```python
from build123d import *

# Parameters (mm, degrees)
BOX002_W          = 10
BOX002_H          = 8
BOX002_DEPTH      = 5
CYLINDER003_R     = 2
CYLINDER003_DEPTH = 10
ARRAY003_X_COUNT  = 5
ARRAY003_X_PITCH  = 10
ARRAY003_Z_COUNT  = 2
ARRAY003_Z_PITCH  = 8
BOX001_W          = 57
BOX001_H          = 2
BOX001_DEPTH      = 22.3


with BuildPart() as cube:
    # Box002 → Box002 (new body)
    with BuildSketch(Plane(origin=(-15, -27, -2.5), x_dir=(1, 0, 0), z_dir=(0, 0, 1))):
        with Locations((5, 4)):
            Rectangle(BOX002_W, BOX002_H)
    extrude(amount=BOX002_DEPTH)


with BuildPart() as array003:
    # Cylinder003 → Cylinder003 (new body)
    with BuildSketch(Plane(origin=(-30, -16, 7), x_dir=(1, 0, 0), z_dir=(0, -1, 0))):
        Circle(CYLINDER003_R)
    extrude(amount=CYLINDER003_DEPTH)

    # Array003 X: Array003 ×5


with BuildPart() as array003_1:
    add(array003.part)
    with Locations(*[(i * ARRAY003_X_PITCH, 0, 0) for i in range(1, ARRAY003_X_COUNT)]):
        add(array003.part)

    # Array003 Z: Array003 ×2


with BuildPart() as array003_2:
    add(array003_1.part)
    with Locations(*[(0, 0, i * ARRAY003_Z_PITCH) for i in range(1, ARRAY003_Z_COUNT)]):
        add(array003_1.part)


with BuildPart() as cut006:
    # Box001 → Box001 (new body)
    with BuildSketch(Plane(origin=(-38.5, -22, 0), x_dir=(1, 0, 0), z_dir=(0, 0, 1))):
        with Locations((28.5, 1)):
            Rectangle(BOX001_W, BOX001_H)
    extrude(amount=BOX001_DEPTH)

    # Cut005: cut Array003
    add(array003_2.part, mode=Mode.SUBTRACT)

    # Cut006: cut Cube
    add(cube.part, mode=Mode.SUBTRACT)


solid = cut006.part
```
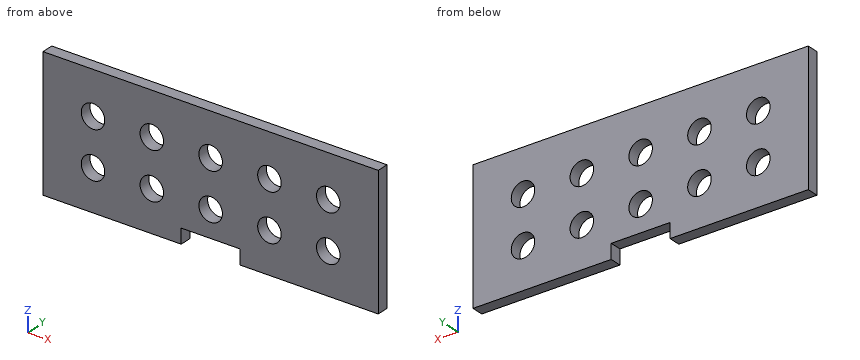
CAD build for the part. Positions are in the model's coordinates, mm. Round coordinates to 2 decimals unless told otherwise and drop trailing zeros. Write each loop counter-clockwise with the first axis right and the second up, starting at its lowest first coordinate (ties: lowest second). Pieces come first, ordered by that corner, then holes. Notation, with made-up numbers: (-23, 1.25) -> (-2, 1.25) arc R14 cw to (-2, 16.25) -> close; hole circle Ø6 at (84.5, 3). An arc over 180 degrees is marked (long way). Answer in a Markdown table with one row per item. Add a question column.
Item 1: Saw through at B-B, the plane y = -20.6. Count the separate pieces of the cut face and the enclosed holes in it, then the cut area to 3 significant figures.
Item 2: Saw through at A-A, the plane z = 15. Write the cut outline in (x, y), then the cut area to 3 significant figures.
Item 3: Saw through at D-D, the plane x = -0.5. Write the cut outline in (y, z).
Item 4: Drop a flat-ended pin along its axis: pin 1 Ø2 at (x, z) = (-20.5, 15) entering from +Y. Give the stop position or say it passes through.
Item 5: Drill centre lines: line 1 (X direction, y = -21.45, z = 15); line 2 (Z direction, x = -20, y = -21.5); line 3 (Z direction, x = -10, y = -20.7). Where is each one in solid material? Low to high. Write a range as from..to.
Item 6: Saw through at C-C, the plane x = -20. Write the cut outline in (y, z), then the cut area to 3 significant figures.
Findings below:
| question | item | result |
|---|---|---|
| 1 | separate pieces | 1 |
| 1 | enclosed holes | 10 |
| 1 | area | 1,120 mm^2 |
| 2 | outline | (-38.5, -22) -> (-32, -22) -> (-32, -20) -> (-38.5, -20) -> close; (-28, -22) -> (-22, -22) -> (-22, -20) -> (-28, -20) -> close; (-18, -22) -> (-12, -22) -> (-12, -20) -> (-18, -20) -> close; (-8, -22) -> (-2, -22) -> (-2, -20) -> (-8, -20) -> close; (2, -22) -> (8, -22) -> (8, -20) -> (2, -20) -> close; (12, -22) -> (18.5, -22) -> (18.5, -20) -> (12, -20) -> close |
| 2 | area | 74.0 mm^2 |
| 3 | outline | (-22, 0) -> (-20, 0) -> (-20, 5.06) -> (-22, 5.06) -> close; (-22, 8.94) -> (-20, 8.94) -> (-20, 13.06) -> (-22, 13.06) -> close; (-22, 16.94) -> (-20, 16.94) -> (-20, 22.3) -> (-22, 22.3) -> close |
| 4 | pin 1 | passes through |
| 5 | line 1 | x = -38.5..-32, -28..-22, -18..-12, -8..-2, 2..8, 12..18.5 |
| 5 | line 2 | z = 0..5, 9..13, 17..22.3 |
| 5 | line 3 | z = 2.5..5, 9..13, 17..22.3 |
| 6 | outline | (-22, 0) -> (-20, 0) -> (-20, 5) -> (-22, 5) -> close; (-22, 9) -> (-20, 9) -> (-20, 13) -> (-22, 13) -> close; (-22, 17) -> (-20, 17) -> (-20, 22.3) -> (-22, 22.3) -> close |
| 6 | area | 28.6 mm^2 |
